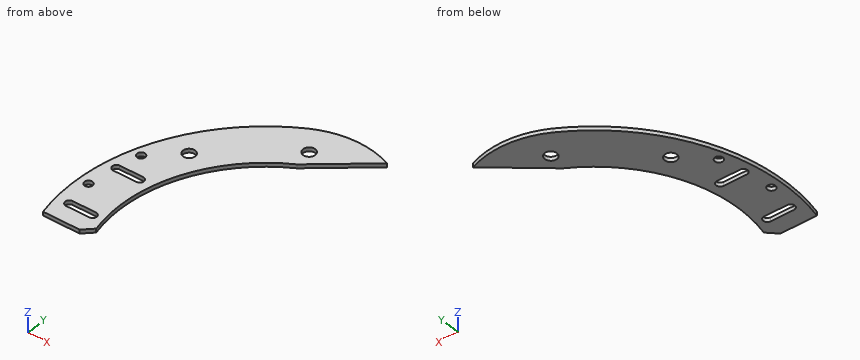
```python
from build123d import *

# Parameters (mm, degrees)
BOSS_EXTRUDE1_DEPTH              = 3.175
CUT_EXTRUDE1_DEPTH               = 3.175
SKETCH4_R                        = 3.302
CUT_EXTRUDE2_DEPTH               = 3.175
F_25_64_0_39063_DIAMETER_HOLE1_D = 9.922002


with BuildPart() as part:
    # Sketch1 → Boss-Extrude1 (new body)
    with BuildSketch(Plane.XY):
        with BuildLine():
            Line((-153.9561854, -36.5125), (-123.978950074, -36.5125))
            Line((-123.978950074, -36.5125), (-116.548747531, -29.082297457))
            ThreePointArc((-116.548747531, -29.082297457), (-110.518418653, 46.73895163), (-59.613700036, 103.253872686))
            Line((-59.613700036, 103.253872686), (-15.834260112, 139.989184579))
            ThreePointArc((-15.834260112, 139.989184579), (-47.43896166, 145.45922618), (-78.234917279, 136.493311135))
            ThreePointArc((-78.234917279, 136.493311135), (-145.12613966, 62.696527677), (-153.9561854, -36.5125))
        make_face()
    extrude(amount=BOSS_EXTRUDE1_DEPTH)

    # Sketch2 → Cut-Extrude1 (cut)
    with BuildSketch(Plane.XY.offset(3.175)):
        with BuildLine():
            Line((-146.3361854, -16.0655), (-127.2861854, -16.0655))
            ThreePointArc((-127.2861854, -16.0655), (-123.9841854, -19.3675), (-127.2861854, -22.6695))
            Line((-127.2861854, -22.6695), (-146.3361854, -22.6695))
            ThreePointArc((-146.3361854, -22.6695), (-149.6381854, -19.3675), (-146.3361854, -16.0655))
        make_face()
        with BuildLine():
            Line((-146.3361854, 31.5595), (-127.2861854, 31.5595))
            ThreePointArc((-127.2861854, 31.5595), (-123.9841854, 28.2575), (-127.2861854, 24.9555))
            Line((-127.2861854, 24.9555), (-146.3361854, 24.9555))
            ThreePointArc((-146.3361854, 24.9555), (-149.6381854, 28.2575), (-146.3361854, 31.5595))
        make_face()
    extrude(amount=-CUT_EXTRUDE1_DEPTH, mode=Mode.SUBTRACT)

    # Sketch4 → Cut-Extrude2 (cut)
    with BuildSketch(Plane.XY.offset(3.175)):
        with Locations((-149.837364131, 4.445)):
            Circle(SKETCH4_R)
        with Locations((-142.427155303, 48.347866959)):
            Circle(SKETCH4_R)
    extrude(amount=-CUT_EXTRUDE2_DEPTH, mode=Mode.SUBTRACT)

    # 25/64 (0.39063) Diameter Hole1 (through all)
    with Locations(Plane.XY.offset(3.175)):
        with Locations((-120.049591928, 69.120810664), (-61.677005362, 118.101226522)):
            Hole(F_25_64_0_39063_DIAMETER_HOLE1_D / 2)


solid = part.part
```
The model under review builds one solid part; all positions refer to its coordinate system, in mm. Give positions to 0.01 mm unless a question says otherwise; leave off trailing zeros. Write each loop counter-clockwise with the first axis right and the second up, starting at its lowest first coordinate (ties: lowest second). Pieces come first, ordered by that corner, then holes. Notation, with made-up numbers: (65, -5) - (89, -5) arc R27 cw to (89, 26) - close; hole circle Ø6 at (63, 37). An arc over 180 degrees is marked (long way). Answer in a Markdown table with one row per item. Add a question column.
1. We need section D-D on x = -136.5. Write out the cut boundary in (y, z) (1 decimal).
2. Wall thickness on line 1 along Y through (x, z) = (-142.5, 0.95); line 2 along Y through (x, z) = (-133.5, 1.5); line 3 along Y through (x, z) = (-129, 0.75): over which ranges is each line inside the solid? List them lowest first. Write a range as [from, to].
3. Insertion check: P1, Ø9, axis at x = -61.68, y = 118.1, coming from the -Z side. The pin has a flat end and moves straight along its axis. Give the tip position at first contact, or say it passes through.
4. We need section B-B on y = 116. Write out the cut boundary in (x, z) (3 decimals), then the cut area to 3 significant figures.
5. We need section C-C on x = -64. Write out the cut boundary in (y, z) (3 decimals), then the cut area to 3 significant figures.
6. We need section A-A on z = 2.25. Write out the cut boundary in (x, y) (1 decimal), then the cut area to 3 significant figures.
Ans:
| question | item | result |
|---|---|---|
| 1 | outline | (-36.5, 0) - (-22.7, 0) - (-22.7, 3.2) - (-36.5, 3.2) - close; (-16.1, 0) - (25, 0) - (25, 3.2) - (-16.1, 3.2) - close; (31.6, 0) - (79.5, 0) - (79.5, 3.2) - (31.6, 3.2) - close |
| 2 | line 1 | y = [-36.51, -22.67], [-16.07, 24.96], [31.56, 45.05], [51.65, 68.38] |
| 2 | line 2 | y = [-36.51, -22.67], [-16.07, 24.96], [31.56, 84.42] |
| 2 | line 3 | y = [-36.51, -22.67], [-16.07, 24.96], [31.56, 91.06] |
| 3 | P1 | passes through |
| 4 | outline | (-106.755, 0) - (-66.171, 0) - (-66.171, 3.175) - (-106.755, 3.175) - close; (-57.183, 0) - (-44.423, 0) - (-44.423, 3.175) - (-57.183, 3.175) - close |
| 4 | area | 169 mm^2 |
| 5 | outline | (100.671, 0) - (113.718, 0) - (113.718, 3.175) - (100.671, 3.175) - close; (122.485, 0) - (142.541, 0) - (142.541, 3.175) - (122.485, 3.175) - close |
| 5 | area | 105 mm^2 |
| 6 | outline | (-154, -36.5) - (-124, -36.5) - (-116.5, -29.1) arc R118.4 cw to (-59.6, 103.3) - (-15.8, 140) arc R71.2 ccw to (-78.2, 136.5) arc R156.5 ccw to start; hole circle Ø6.6 at (-149.8, 4.4); hole (-146.3, -22.7) - (-127.3, -22.7) arc R3.3 ccw to (-127.3, -16.1) - (-146.3, -16.1) arc R3.3 ccw to start; hole (-146.3, 25) - (-127.3, 25) arc R3.3 ccw to (-127.3, 31.6) - (-146.3, 31.6) arc R3.3 ccw to start; hole circle Ø6.6 at (-142.4, 48.3); hole circle Ø9.9 at (-120, 69.1); hole circle Ø9.9 at (-61.7, 118.1) |
| 6 | area | 7,750 mm^2 |
